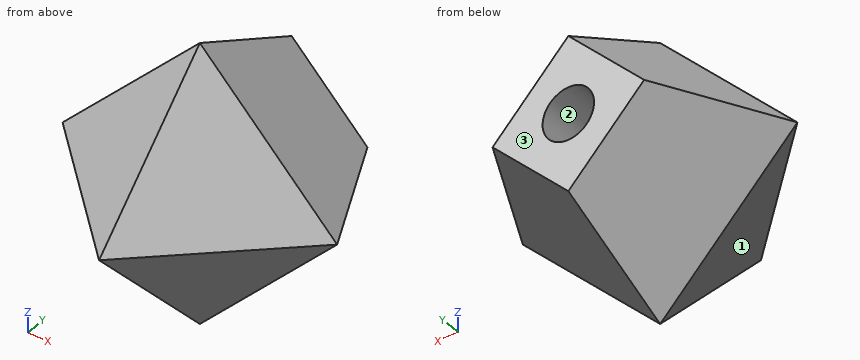
```python
from build123d import *

# Parameters (mm, degrees)
BOSS_EXTRUDE1_DEPTH = 25.4
SKETCH2_W           = 48.842738796
SKETCH2_H           = 57.963308492
CUT_EXTRUDE1_DEPTH  = 25.4
CIRPATTERN1_COUNT   = 4
BOSS_EXTRUDE2_DEPTH = 25.4
SKETCH4_W           = 55.511744094
SKETCH4_H           = 37.462262811
CUT_EXTRUDE2_DEPTH  = 25.4
CIRPATTERN2_COUNT   = 4
SKETCH5_R           = 4.7625
CUT_EXTRUDE3_DEPTH  = 25.4


with BuildPart() as part:
    # Sketch1 → Boss-Extrude1 (new body)
    with BuildSketch(Plane.XY):
        Polygon((64.875616583, 27.293462823), (90.275616583, 27.293462823), (90.275616583, 49.518462823), (76.253828643, 49.518462823), align=None)
    boss_extrude1 = extrude(amount=BOSS_EXTRUDE1_DEPTH)

    # Sketch2 → Cut-Extrude1 (cut)
    with BuildSketch(Plane(origin=(22.502369916, -11.520213127, -22.502369916), x_dir=(0.7469488589136901, 0.3029911037986301, 0.5918308822513607), z_dir=(-0.664881494830121, 0.3403897702119252, 0.6648814948301214))):
        with Locations((74.048071209, 28.981654246)):
            Rectangle(SKETCH2_W, SKETCH2_H)
    cut_extrude1 = extrude(amount=CUT_EXTRUDE1_DEPTH, mode=Mode.SUBTRACT)

    # CirPattern1: Boss-Extrude1, Cut-Extrude1 ×4 about axis
    cirpattern1_axis = Axis((90.275616583, 0, 0), (0, 1, 0))
    add([boss_extrude1.rotate(cirpattern1_axis, i * 360 / CIRPATTERN1_COUNT) for i in range(1, CIRPATTERN1_COUNT)])
    add([cut_extrude1.rotate(cirpattern1_axis, i * 360 / CIRPATTERN1_COUNT) for i in range(1, CIRPATTERN1_COUNT)], mode=Mode.SUBTRACT)

    # Sketch3 → Boss-Extrude2 (add)
    with BuildSketch(Plane.XY):
        Polygon((90.275616583, 27.293462823), (64.875616583, 27.293462823), (90.275616583, 2.897951184), align=None)
    boss_extrude2 = extrude(amount=BOSS_EXTRUDE2_DEPTH)

    # Sketch4 → Cut-Extrude2 (cut)
    with BuildSketch(Plane(origin=(30.250165476, 31.49571997, -30.250165476), x_dir=(0.822040500476201, -0.41068588128331385, 0.3944445746760687), z_dir=(0.5694290259346084, 0.5928753400558371, -0.56942902593461))):
        with Locations((65.735556872, -20.321660951)):
            Rectangle(SKETCH4_W, SKETCH4_H)
    cut_extrude2 = extrude(amount=-CUT_EXTRUDE2_DEPTH, mode=Mode.SUBTRACT)

    # CirPattern2: Boss-Extrude2, Cut-Extrude2 ×4 about axis
    cirpattern2_axis = Axis((90.275616583, 0, 0), (0, 1, 0))
    add([boss_extrude2.rotate(cirpattern2_axis, i * 360 / CIRPATTERN2_COUNT) for i in range(1, CIRPATTERN2_COUNT)])
    add([cut_extrude2.rotate(cirpattern2_axis, i * 360 / CIRPATTERN2_COUNT) for i in range(1, CIRPATTERN2_COUNT)], mode=Mode.SUBTRACT)

    # Sketch5 → Cut-Extrude3 (cut)
    with BuildSketch(Plane(origin=(0, 49.518462823, 0), x_dir=(1, 0, 0), z_dir=(0, 1, 0))):
        with Locations(Location((90.275616583, 0, 0), (0, 0, 270))):
            Circle(SKETCH5_R)
    extrude(amount=-CUT_EXTRUDE3_DEPTH, mode=Mode.SUBTRACT)


solid = part.part
```
The model under review builds one solid part; all positions refer to its coordinate system, in mm. Face numbers are marked on the shaded views. Round coordinates to 2 decimals unless told otherwise and drop trailing zeros. Loops run counter-clockwise (first coordinate to the right, second up) from the corner with the lowest first, then second, coordinate; pieces in that order, holes last. Notation, with made-up numbers: (-12, 86) - (32, 86) arc R21 cw to (32, 101) - close; hole circle Ø6 at (11, 11.5). An arc over 180 degrees is marked (long way). Use a Markdown table: item, result. Add a question column.
Q1. The part is to be moulded in two halves that separate along Z. For the marked faces 1, 2 and 3, say which applies: pulls with the +Z half, pulls with the -Z half, needs draft (parallel to the pull), parting line crosses it, or undercut.
Q2. Add section B-B (z = 4). State the section outline as (x, y) points.
Q3. For probe 1 along X at (y, z) = (31, -3.5); probe 2 along X at (y, z) = (29, -3); probe 3 along Z at (x, y) = (88.5, 23), list the stretches that pass through material, from the lowest coordinate up.
Q4. Add section C-C (x = 100.5). State the section outline as (y, z) points, plus the area to 3 significant figures.
Q5. Insertion check: pin 1 Ø2 at (y, z) = (40.5, 14.5) entering from -X; pin 2 Ø3 at (x, z) = (89, 1.5) entering from +Y; pin 3 Ø6 at (y, z) = (31.5, 4.5) entering from +X; pin 4 Ø1 at (y, z) = (43.5, 18) entering from +X. Each pin has a flat end and moves straight along its axis. Give the tip position at first contact, or say it passes through.
Q6. Add section D-D (z = -13). State the section outline as (x, y) points.
Q7. Add section A-A (y = 25). State the section outline as (x, z) points (1 decimal).
Worked answers:
| question | item | result |
|---|---|---|
| 1 | face 1 | pulls with the -Z half |
| 1 | face 2 | undercut |
| 1 | face 3 | needs draft |
| 2 | outline | (68.88, 27.29) - (90.28, 6.74) - (111.68, 27.29) - (100.3, 49.52) - (92.86, 49.52) - (92.86, 24.12) - (87.69, 24.12) - (87.69, 49.52) - (80.25, 49.52) - close |
| 3 | probe 1 | 70.27 to 87.05, 93.51 to 110.28 |
| 3 | probe 2 | 68.75 to 86.58, 93.97 to 111.8 |
| 3 | probe 3 | -19.15 to 19.15 |
| 4 | outline | (12.72, 0) - (27.29, -15.18) - (49.52, -3.8) - (49.52, 3.8) - (27.29, 15.18) - close |
| 4 | area | 643 mm² |
| 5 | pin 1 | x = 85.01 |
| 5 | pin 2 | y = 24.12 |
| 5 | pin 3 | x = 112.39 |
| 5 | pin 4 | through |
| 6 | outline | (77.88, 27.29) - (90.28, 15.38) - (102.68, 27.29) - (91.3, 49.52) - (89.25, 49.52) - close |
| 7 | outline | (67.3, 0) - (90.3, -23) - (113.3, 0) - (90.3, 23) - close; hole circle Ø9.5 at (90.3, 0) |
